Input: part model. Units: mm. Frame: model coordinates. Give positions to 0.01 mm unless a question says otherwise; leave off trailing zeros. Loops run counter-clockwise (first coordinate to the right, second up) from the corner with the lowest first, then second, coordinate; pieces in that order, holes last. Notation, with made-up numbers: (27, 5.25) -> (62, 5.25) arc R16 cw to (62, 10.25) -> close; hole circle Ø11 at (3, -9). An arc over 180 degrees is marked (long way). Use CSV: the item, a comma, the result in double quotes.
Autodesk Inventor part; units mm, degrees
ref_plane "YZ Plane" through (0, 0, 0) normal (1, 0, 0) x (0, 1, 0)
ref_plane "XZ Plane" through (0, 0, 0) normal (0, 1, 0) x (-1, 0, 0)
ref_plane "XY Plane" through (0, 0, 0) normal (0, 0, 1) x (1, 0, 0)
ref_plane "Arbeitsebene1" through (0, 0, 0.5) normal (0, 0, 1) x (1, 0, 0)
sketch "Skizze1" plane through (0, 0, 0.5) normal (0, 0, 1) x (1, 0, 0)
  circle A0 centre (12, 2.9) radius 1.5
  circle A1 centre (-12, 2.9) radius 1.5
  line L0 (2.5, 12.9) -> (2.5, -7.1)
  line L1 (2.5, -7.1) -> (2.25, -7.1)
  line L2 (2.25, -7.1) -> (2, -7.1)
  line L3 (2, -7.1) -> (1.75, -7.1)
  line L4 (1.75, -7.1) -> (1.5, -7.1)
  line L5 (1.5, -7.1) -> (1.25, -7.1)
  line L6 (1.25, -7.1) -> (1, -7.1)
  line L7 (1, -7.1) -> (0.75, -7.1)
  line L8 (0.75, -7.1) -> (0.5, -7.1)
  line L9 (0.5, -7.1) -> (0.25, -7.1)
  line L10 (0.25, -7.1) -> (0, -7.1)
  line L11 (0, -7.1) -> (-0.25, -7.1)
  line L12 (-0.25, -7.1) -> (-0.5, -7.1)
  line L13 (-0.5, -7.1) -> (-0.75, -7.1)
  line L14 (-0.75, -7.1) -> (-1, -7.1)
  line L15 (-1, -7.1) -> (-1.25, -7.1)
  line L16 (-1.25, -7.1) -> (-1.5, -7.1)
  line L17 (-1.5, -7.1) -> (-1.75, -7.1)
  line L18 (-1.75, -7.1) -> (-2, -7.1)
  line L19 (-2, -7.1) -> (-2.25, -7.1)
  line L20 (-2.25, -7.1) -> (-2.5, -7.1)
  line L21 (-2.5, -7.1) -> (-2.5, 12.9)
  line L22 (-2.5, 12.9) -> (-38, 12.9)
  line L23 (-38, 12.9) -> (-38, -12.9)
  line L24 (-38, -12.9) -> (38, -12.9)
  line L25 (38, -12.9) -> (38, 12.9)
  line L26 (38, 12.9) -> (2.5, 12.9)
  line L27 (25, -11) -> (-25, -11)
  line L28 (-25, -11) -> (-25, 11)
  line L29 (-25, 11) -> (25, 11)
  line L30 (25, 11) -> (25, -11)
  line L31 (25, -11) -> (-25, 11) construction
  line L32 (-25, -11) -> (25, 11) construction
  point P0 (0, 0)
  point P1 (-2.5, 11)
  point P2 (2.5, 11)
  dimension "d0" = 50
  dimension "d1" = 22
extrude "Extrusion1" add sketch "Skizze1" along normal blind 0.15 contours A0 | A1 | L29 L30 L27 L28 L21 L20 L19 L18 L17 L16 L15 L14 L13 L12 L11 L10 L9 L8 L7 L6 L5 L4 L3 L2 L1 L0
properties part number "00_coverglass_50x22"
1) Section query C-C (x = 1.5). Return loops of the section in (y, z), then the cut area to 3 significant figures.
From the geometry:
outline,"(-11, 0.5) -> (-7.1, 0.5) -> (-7.1, 0.65) -> (-11, 0.65) -> close"
area,"0.585 mm^2"
2) Section query A-A (y = -6). Return loops of the section in (x, z).
From the geometry:
outline,"(-25, 0.5) -> (-2.5, 0.5) -> (-2.5, 0.65) -> (-25, 0.65) -> close; (2.5, 0.5) -> (25, 0.5) -> (25, 0.65) -> (2.5, 0.65) -> close"
3) Section query B-B (z = 0.6). Return loops of the section in (x, y), then the cut area to 3 significant figures.
From the geometry:
outline,"(-25, -11) -> (25, -11) -> (25, 11) -> (2.5, 11) -> (2.5, -7.1) -> (-2.5, -7.1) -> (-2.5, 11) -> (-25, 11) -> close"
area,"1,010 mm^2"
4) Ray query, line 1 (X direction, y = 2.5, z = 0.6). Return the intervals inside material, ascending.
From the geometry:
line 1,"x = -25 to -2.5, 2.5 to 25"
